Input: part model. Units: mm. Frame: model coordinates. Face numbers are marked on the shaded views. Coordinates: 2 decimals unless noted, no trailing zeros. Write each loop counter-clockwise with the first axis right and the second up, starting at its lowest first coordinate (ties: lowest second). Pieces come first, ordered by that corner, then holes.
1) Line query: L1, parallel to Z at x = -114, y = -53.5; L2, parallel to X at y = -38.5, z = 78; L3, parallel to Z at x = -129.5, y = -38. Output: solid intervals per line, ascending.
2) Pin query (flat end, axial travel): pin 1 Ø12 at (y, z) = (-55, 76.5) entering from -X; pin 2 Ø18 at (x, y) = (-112.5, -38.5) entering from -Z; pin 3 Ø3 at (y, z) = (-54, 38.5) entering from -X; pin 4 Ø2 at (x, z) = (-112.5, 49.5) entering from -Y. Return the tip coordinate at first contact, or that it passes through.
3) Section query A-A (z = 64.5). Output: boundary loops of the cut face in (x, y).
4) Draft query along Y for the marked faces 1, 2 and 3. Return one class per face: pulls with the +Y half, pulls with the -Y half, needs draft (parallel to the pull), parting line crosses it, or undercut.
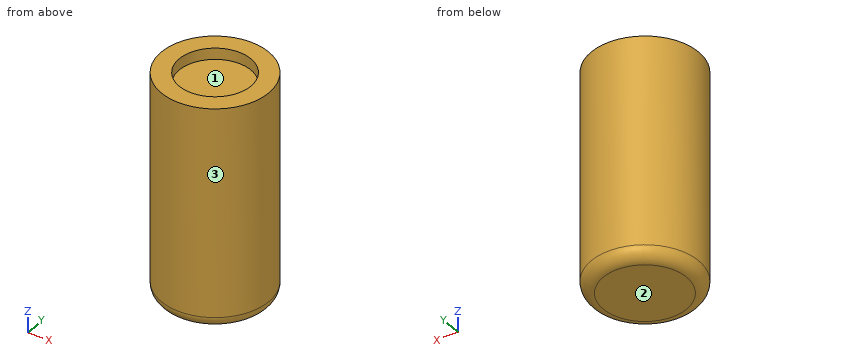
from build123d import *

# Parameters (mm, degrees)
F0_R     = 22.8092
F1_DEPTH = 93.599
F2_R     = 15.24
F3_DEPTH = 4.7752
F4_R     = 5.08
F5_T     = -2.54


with BuildPart() as f1:
    # F0 (on Top) → F1 (new body)
    with BuildSketch(Plane.XY):
        with Locations((-112.9804104567, -38.8761870563)):
            Circle(F0_R)
    extrude(amount=F1_DEPTH)

    # F2 (on face) → F3 (cut)
    with BuildSketch(Plane.XY.offset(93.599)):
        with Locations((-112.9804104567, -38.8761870563)):
            Circle(F2_R)
    extrude(amount=-F3_DEPTH, mode=Mode.SUBTRACT)

    # F4
    f4_edges = [f1.edges().sort_by_distance(p)[0] for p in [
        (-135.78961, -38.876187, 0),
    ]]
    fillet(f4_edges, radius=F4_R)

    # F5 (hollow: no face is removed)
    offset(amount=F5_T, kind=Kind.INTERSECTION, mode=Mode.SUBTRACT)


solid = f1.part
Answer:
1. L1: z = 0 to 2.54, 86.28 to 88.82
1. L2: x = -135.79 to -133.25, -92.71 to -90.17
1. L3: z = 0 to 2.54, 86.28 to 93.6
2. pin 1: stops at x = -133.42
2. pin 2: stops at z = 0
2. pin 3: stops at x = -131.27
2. pin 4: stops at y = -61.69
3. outline: circle Ø45.62 at (-112.98, -38.88); hole circle Ø40.54 at (-112.98, -38.88)
4. face 1: undercut
4. face 2: needs draft
4. face 3: parting line crosses it
